Could you check a few things on this model? Use its own coordinates, in mm. Face numbers are marked on the shaded views. A direction names the side the tool comes from. Round coordinates to 2 decimals unless told otherwise and drop trailing zeros. Write each loop counter-clockwise with the first axis right and the second up, starting at its lowest first coordinate (ties: lowest second). Pieces come first, ordered by that corner, then holes. Notation, with made-up numbers: (46, 62) - (87, 62) arc R31 ccw to (87, 93) - close; hole circle Ø10 at (47.25, 44.5). An arc over 180 degrees is marked (long way). Write each question's results on one line, items separated by ' | '. Start each with the question number.
(1) Thinking about a two-plate mould opening in Z: for the marked faces 1, 2 and 3, which applies, +Z half, -Z half, draft (parallel to the pull), parting line (faces both ways), or undercut?
(2) Imagine slicing it at D-D on x = 5. Write out the boundary of the cut face in (y, z), then the cut area to 3 significant figures.
(3) Please list where these lines run through material, in increasing order: line 1 (X direction, y = 33, z = 2); line 2 (X direction, y = 7, z = -3); line 3 (Z direction, x = -16.5, y = 24). Write a range as [from, to].
(4) On a 3-axis mill with a long thin cutter (end or side, diameter ignored), from which of +Z, -Z, +X, -X, +Y, -Y can I reach the whole of each face in a straight line? I mean the marked faces 4 and 5. Say none if no direction works.
(5) Imagine slicing it at B-B on x = 66. Write out the boundary of the cut face in (y, z), then the cut area to 3 significant figures.
(6) For P1, Ø2.5, axis at x = -15, y = 24.5, coming from the -Z side; P2, Ø5, axis at y = 24.5, z = -0.5, coming from the -X side; P3, Ø1, axis at y = 20.5, z = 19, coming from the -X side, each with a flat end and sliding along its axis, tell me the tip position at first contact or that it passes through.
(7) Imagine slicing it at A-A on z = 4.5. Write out the boundary of the cut face in (x, y).
(8) Imagine slicing it at C-C on y = 3. Write out the boundary of the cut face in (x, z).
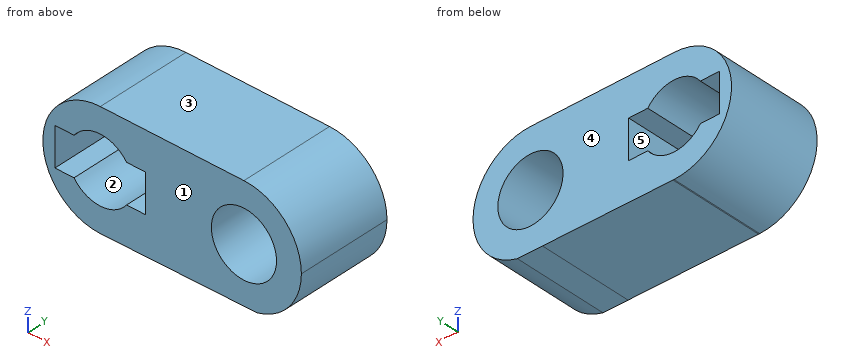
```python
from build123d import *

# Parameters (mm, degrees)
F0_R     = 14.4101824993
F1_DEPTH = 41.91
F4_DEPTH = 119.38


# Not quite as in the source:
# - a feature of the source that left no trace in its solid (it failed there, or was rolled back) is left out


with BuildPart() as f1:
    # F0 (on Front) → F1 (new body)
    with BuildSketch(Plane.XZ):
        with BuildLine():
            ThreePointArc((0.4902951327, -25.3952674859), (18.133029206, -17.7863220429), (25.4, 0))
            ThreePointArc((25.4, 0), (17.9605122421, 17.9605122421), (0, 25.4))
            ThreePointArc((0, 25.4), (-25.4, 0), (0, -25.4))
            Line((0, -25.4), (0.4902951327, -25.3952674859))
        make_face()
        with BuildLine():
            ThreePointArc((-11.6233856549, 8.5176443681), (0, 14.4101824993), (11.6233856549, 8.5176443681))
            Line((11.6233856549, 8.5176443681), (20.0593080372, 8.5176443681))
            Line((20.0593080372, 8.5176443681), (20.0593080372, -8.5176443681))
            Line((20.0593080372, -8.5176443681), (11.6233856549, -8.5176443681))
            ThreePointArc((11.6233856549, -8.5176443681), (0, -14.4101824993), (-11.6233856549, -8.5176443681))
            Line((-11.6233856549, -8.5176443681), (-20.0593080372, -8.5176443681))
            Line((-20.0593080372, -8.5176443681), (-20.0593080372, 8.5176443681))
            Line((-20.0593080372, 8.5176443681), (-11.6233856549, 8.5176443681))
        make_face(mode=Mode.SUBTRACT)
        with BuildLine():
            ThreePointArc((0, 25.4), (17.9605122421, 17.9605122421), (25.4, 0))
            ThreePointArc((25.4, 0), (18.133029206, -17.7863220429), (0.4902951327, -25.3952674859))
            Line((0.4902951327, -25.3952674859), (58.1880762297, -24.8383466813))
            ThreePointArc((58.1880762297, -24.8383466813), (38.2408035984, 2.670767146), (63.5, 25.4))
            Line((63.5, 25.4), (0, 25.4))
        make_face()
        with BuildLine():
            ThreePointArc((88.9, 0), (81.4605122421, 17.9605122421), (63.5, 25.4))
            ThreePointArc((63.5, 25.4), (38.2408035984, 2.670767146), (58.1880762297, -24.8383466813))
            Line((58.1880762297, -24.8383466813), (69.2903876179, -24.7311829728))
            ThreePointArc((69.2903876179, -24.7311829728), (83.4027114421, -15.7810670505), (88.9, 0))
        make_face()
        with Locations((63.5, 0)):
            Circle(F0_R, mode=Mode.SUBTRACT)
        with Locations((63.5, 0)):
            Circle(F0_R)
        with BuildLine():
            ThreePointArc((-11.6233856549, -8.5176443681), (-14.4101824993, 0), (-11.6233856549, 8.5176443681))
            Line((-11.6233856549, 8.5176443681), (-20.0593080372, 8.5176443681))
            Line((-20.0593080372, 8.5176443681), (-20.0593080372, -8.5176443681))
            Line((-20.0593080372, -8.5176443681), (-11.6233856549, -8.5176443681))
        make_face()
        with BuildLine():
            ThreePointArc((11.6233856549, -8.5176443681), (13.6957743156, -4.4809737288), (14.4101824993, 0))
            ThreePointArc((14.4101824993, 0), (13.6957743156, 4.4809737288), (11.6233856549, 8.5176443681))
            Line((11.6233856549, 8.5176443681), (-11.6233856549, 8.5176443681))
            ThreePointArc((-11.6233856549, 8.5176443681), (-14.4101824993, 0), (-11.6233856549, -8.5176443681))
            Line((-11.6233856549, -8.5176443681), (11.6233856549, -8.5176443681))
        make_face()
        with BuildLine():
            Line((-11.6233856549, 8.5176443681), (11.6233856549, 8.5176443681))
            ThreePointArc((11.6233856549, 8.5176443681), (0, 14.4101824993), (-11.6233856549, 8.5176443681))
        make_face()
        with BuildLine():
            ThreePointArc((-11.6233856549, -8.5176443681), (0, -14.4101824993), (11.6233856549, -8.5176443681))
            Line((11.6233856549, -8.5176443681), (-11.6233856549, -8.5176443681))
        make_face()
        with BuildLine():
            ThreePointArc((11.6233856549, 8.5176443681), (13.6957743156, 4.4809737288), (14.4101824993, 0))
            ThreePointArc((14.4101824993, 0), (13.6957743156, -4.4809737288), (11.6233856549, -8.5176443681))
            Line((11.6233856549, -8.5176443681), (20.0593080372, -8.5176443681))
            Line((20.0593080372, -8.5176443681), (20.0593080372, 8.5176443681))
            Line((20.0593080372, 8.5176443681), (11.6233856549, 8.5176443681))
        make_face()
    extrude(amount=-F1_DEPTH)

    # F0 (on Front) → F4 (cut)
    with BuildSketch(Plane.XZ):
        with BuildLine():
            ThreePointArc((-11.6233856549, -8.5176443681), (-14.4101824993, 0), (-11.6233856549, 8.5176443681))
            Line((-11.6233856549, 8.5176443681), (-20.0593080372, 8.5176443681))
            Line((-20.0593080372, 8.5176443681), (-20.0593080372, -8.5176443681))
            Line((-20.0593080372, -8.5176443681), (-11.6233856549, -8.5176443681))
        make_face()
        with BuildLine():
            Line((-11.6233856549, 8.5176443681), (11.6233856549, 8.5176443681))
            ThreePointArc((11.6233856549, 8.5176443681), (0, 14.4101824993), (-11.6233856549, 8.5176443681))
        make_face()
        with BuildLine():
            ThreePointArc((11.6233856549, 8.5176443681), (13.6957743156, 4.4809737288), (14.4101824993, 0))
            ThreePointArc((14.4101824993, 0), (13.6957743156, -4.4809737288), (11.6233856549, -8.5176443681))
            Line((11.6233856549, -8.5176443681), (20.0593080372, -8.5176443681))
            Line((20.0593080372, -8.5176443681), (20.0593080372, 8.5176443681))
            Line((20.0593080372, 8.5176443681), (11.6233856549, 8.5176443681))
        make_face()
        with BuildLine():
            ThreePointArc((11.6233856549, -8.5176443681), (13.6957743156, -4.4809737288), (14.4101824993, 0))
            ThreePointArc((14.4101824993, 0), (13.6957743156, 4.4809737288), (11.6233856549, 8.5176443681))
            Line((11.6233856549, 8.5176443681), (-11.6233856549, 8.5176443681))
            ThreePointArc((-11.6233856549, 8.5176443681), (-14.4101824993, 0), (-11.6233856549, -8.5176443681))
            Line((-11.6233856549, -8.5176443681), (11.6233856549, -8.5176443681))
        make_face()
        with BuildLine():
            ThreePointArc((-11.6233856549, -8.5176443681), (0, -14.4101824993), (11.6233856549, -8.5176443681))
            Line((11.6233856549, -8.5176443681), (-11.6233856549, -8.5176443681))
        make_face()
        with Locations((63.5, 0)):
            Circle(F0_R)
    extrude(amount=-F4_DEPTH, mode=Mode.SUBTRACT)


solid = f1.part
```
Response:
1) face 1: draft | face 2: undercut | face 3: +Z half
2) outline: (0, -25.35) - (41.91, -25.35) - (41.91, -13.51) - (0, -13.51) - close; (0, 13.51) - (41.91, 13.51) - (41.91, 25.4) - (0, 25.4) - close | area: 994 mm²
3) line 1: [-25.32, -20.06], [20.06, 49.23], [77.77, 88.82] | line 2: [-25.22, -20.06], [20.06, 49.41], [77.59, 88.72] | line 3: [-19.31, -8.52], [8.52, 19.31]
4) face 4: +Z, -Z, +X, -X, +Y | face 5: +Y, -Y
5) outline: (0, -24.76) - (41.91, -24.76) - (41.91, -14.19) - (0, -14.19) - close; (0, 14.19) - (41.91, 14.19) - (41.91, 25.28) - (0, 25.28) - close | area: 908 mm²
6) P1: z = -21.36 | P2: x = -25.4 | P3: x = -17.4
7) outline: (-25, 0) - (-20.06, 0) - (-20.06, 41.91) - (-25, 41.91) - close; (20.06, 0) - (49.81, 0) - (49.81, 41.91) - (20.06, 41.91) - close; (77.19, 0) - (88.5, 0) - (88.5, 41.91) - (77.19, 41.91) - close
8) outline: (0, -25.4) - (69.29, -24.73) arc R25.4 ccw to (63.5, 25.4) - (0, 25.4) arc R25.4 ccw to start; hole (-20.06, -8.52) - (-11.62, -8.52) arc R14.41 ccw to (11.62, -8.52) - (20.06, -8.52) - (20.06, 8.52) - (11.62, 8.52) arc R14.41 ccw to (-11.62, 8.52) - (-20.06, 8.52) - close; hole circle Ø28.82 at (63.5, 0)
